Autodesk Inventor part; units mm, degrees
ref_plane "YZ Plane" through (0, 0, 0) normal (1, 0, 0) x (0, 1, 0)
ref_plane "XZ Plane" through (0, 0, 0) normal (0, 1, 0) x (-1, 0, 0)
ref_plane "XY Plane" through (0, 0, 0) normal (0, 0, 1) x (1, 0, 0)
sketch "Esboço1" plane through (0, 0, 0) normal (0, 0, 1) x (1, 0, 0)
  line L0 (-185.5, 0) -> (185.5, 0) construction
  line L1 (0, -112) -> (0, 112) construction
  line L2 (-132.5, 80) -> (132.5, 80)
  line L3 (132.5, 80) -> (132.5, -80)
  line L4 (132.5, -80) -> (-132.5, -80)
  line L5 (-132.5, -80) -> (-132.5, 80)
  line L6 (-125, 80) -> (-125, -80) construction
  line L7 (125, 80) -> (125, -80) construction
  line L8 (125, 12.5) -> (125, -12.5) construction
  line L9 (125, 62.64) -> (125, 37.64) construction
  line L10 (125, 12.5) -> (125, -12.5) construction
  line L11 (125, -64.333) -> (125, -39.333) construction
  circle A0 centre (-107.5, -65) radius 10
  circle A1 centre (107.5, -65) radius 10
  circle A2 centre (-107.5, 65) radius 10
  circle A3 centre (107.5, 65) radius 10
  point P0 (0, 0)
  point P1 (-125, 12.5)
  point P2 (-125, -12.5)
  point P3 (125, 0)
  point P4 (125, 50.14)
  point P5 (125, -51.833)
  point P6 (125, 0)
  point P7 (-95, -50)
  point P8 (-95, 50)
  point P9 (95, -50)
  point P10 (95, 50)
  dimension "d0" = 265
  dimension "d1" = 160
  dimension "d3" = 25
  dimension "d5" = 250
  dimension "d6" = 50.14
  dimension "d16" = 51.833
  dimension "d18" = 20
  dimension "d19" = 25
  dimension "d20" = 15
  dimension "d28" = 100
  dimension "d29" = 190
extrude "Extrusão1" add sketch "Esboço1" along normal blind 10 contours L2 L3 L4 L5 | A0 | A1 | A2 | A3
hole "Furo1" at (-125, 12.5, 0) at (-125, -12.5, 0) at (125, -12.5, 0) at (125, 12.5, 0) at (125, 37.64, 0) at (125, 62.64, 0) at (125, -64.333, 0) at (125, -39.333, 0) direction (0, 0, 1) diameter 4.5 end through all counterbore diameter 8 counterbore depth 4.6
hole "Furo2" at (-107.5, -65, 0) at (107.5, -65, 0) at (107.5, 65, 0) at (-107.5, 65, 0) direction (0, 0, 1) diameter 3.242 end through all
sketch "Esboço2" plane through (0, 0, 10) normal (0, 0, 1) x (1, 0, 0)
  point P0 (0, 0)
  point P1 (-95, -50)
  point P2 (-95, 50)
  point P3 (95, -50)
  point P4 (95, 50)
hole "Furo3" at (-95, -50, 10) at (-95, 50, 10) at (95, -50, 10) at (95, 50, 10) direction (0, 0, -1) diameter 5.5 end through all counterbore diameter 10 counterbore depth 5.7
fillet "Arredondamento1" radius 0.5 4 edges at (-132.5, -80, 5) (-132.5, 80, 5) (132.5, 80, 5) (132.5, -80, 5)
properties part number "GRJ-03-113" material "Fenolite OR"
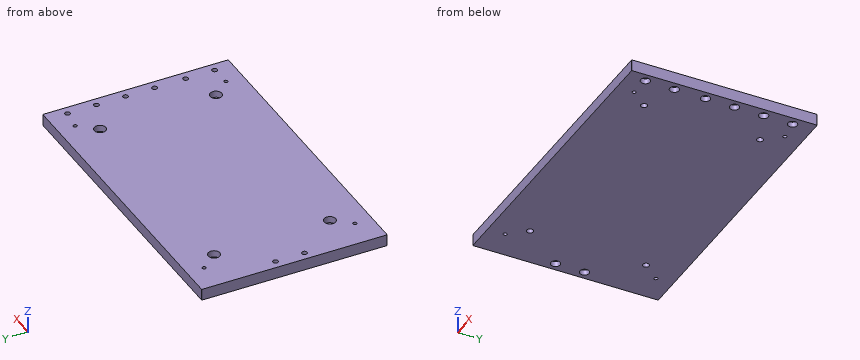
The listing builds one solid part. Answer for the finished solid, in the listing's coordinates (mm). Coordinates: 2 decimals unless noted, no trailing zeros. Order: outer loops, then holes, each group sorted by start corner. A loop starts at its lowest first (then second) coordinate and runs counter-clockwise, first axis right, second up. Notation, with made-up numbers: (-33, -4) -> (-6, -4) arc R10 cw to (-6, 13) -> close; hole circle Ø10 at (-34.75, -19.75). An arc over 180 degrees is marked (long way). Answer in a Markdown table with one row per item. Add a question column.
Item 1: Find section B-B (x = 95). Write down the section's boundary in (y, z), then the cut area to 3 significant figures.
Item 2: Find the intervals of material crossed by L1, parallel to X at y = 12.5, z = 3.3; L2, parallel to X at y = -12.5, z = 6.9; L3, parallel to Y at x = -95, z = 2.5, in increasing order. Write a range as from..to.
Item 3: Each of these flat-tipped pins is pushed along its axis until it touches: P1, Ø2, axis at x = 18, y = 24.5, coming from the -Z side; P2, Ø7, axis at x = 125, y = 62.64, coming from the -Z side; P3, Ø6, axis at x = -95, y = 50, coming from the +Z side. Where does it stop, or does it pass through?
Item 4: Find section A-A (y = -50). Write down the section's boundary in (x, z).
Result set:
| question | item | result |
|---|---|---|
| 1 | outline | (-80, 0) -> (-52.75, 0) -> (-52.75, 4.3) -> (-55, 4.3) -> (-55, 10) -> (-80, 10) -> close; (-47.25, 0) -> (47.25, 0) -> (47.25, 4.3) -> (45, 4.3) -> (45, 10) -> (-45, 10) -> (-45, 4.3) -> (-47.25, 4.3) -> close; (52.75, 0) -> (80, 0) -> (80, 10) -> (55, 10) -> (55, 4.3) -> (52.75, 4.3) -> close |
| 1 | area | 1,440 mm² |
| 2 | L1 | x = -132.5..-129, -121..121, 129..132.5 |
| 2 | L2 | x = -132.5..-127.25, -122.75..122.75, 127.25..132.5 |
| 2 | L3 | y = -80..-52.75, -47.25..47.25, 52.75..80 |
| 3 | P1 | stops at z = 0 |
| 3 | P2 | stops at z = 4.6 |
| 3 | P3 | stops at z = 4.3 |
| 4 | outline | (-132.5, 0) -> (-97.75, 0) -> (-97.75, 4.3) -> (-100, 4.3) -> (-100, 10) -> (-132.5, 10) -> close; (-92.25, 0) -> (92.25, 0) -> (92.25, 4.3) -> (90, 4.3) -> (90, 10) -> (-90, 10) -> (-90, 4.3) -> (-92.25, 4.3) -> close; (97.75, 0) -> (132.5, 0) -> (132.5, 10) -> (100, 10) -> (100, 4.3) -> (97.75, 4.3) -> close |
